For this review, take the finished solid that the model builds, in its own axes (mm). A direction names the side the tool comes from. Round coordinates to 2 decimals unless told otherwise and drop trailing zeros. Order: outer loops, then holes, each group sorted by start corner. A loop starts at its lowest first (then second) coordinate and runs counter-clockwise, first axis right, second up. Notation, with made-up numbers: M -11,11 L 26,11 A24 cw 26,24 Z; hole C 45,63 d4. An arc over 180 degrees is marked long. Use a Markdown table: item, result.
from build123d import *

# Parameters (mm, degrees)
F0_W     = 180.379
F0_H     = 84
F0_W_2   = 176.379
F0_H_2   = 80
F1_DEPTH = 11
F0_W_3   = 164
F0_H_3   = 61
F0_W_4   = 27.5
F0_H_4   = 16
F2_DEPTH = 2
F3_SIZE  = 2


with BuildPart() as f1:
    # F0 (on Top) → F1 (new body)
    with BuildSketch(Plane.XY):
        with Locations((-90.1895, 42)):
            Rectangle(F0_W, F0_H)
        with Locations((-90.1895, 42)):
            Rectangle(F0_W_2, F0_H_2, mode=Mode.SUBTRACT)
    extrude(amount=F1_DEPTH)

    # F0 (on Top) → F2 (join)
    with BuildSketch(Plane.XY):
        with Locations((-90.1895, 42)):
            Rectangle(F0_W_2, F0_H_2)
        with Locations((-91.379, 38.431)):
            Rectangle(F0_W_3, F0_H_3, mode=Mode.SUBTRACT)
        with Locations((-91.379, 38.431)):
            Rectangle(F0_W_3, F0_H_3)
        with BuildLine():
            ThreePointArc((-170.879, 64.931), (-171.9396601718, 67.4916601718), (-169.379, 66.431))
            Line((-169.379, 66.431), (-13.379, 66.431))
            ThreePointArc((-13.379, 66.431), (-11.879, 67.931), (-10.379, 66.431))
            ThreePointArc((-10.379, 66.431), (-10.8183398282, 65.3703398282), (-11.879, 64.931))
            Line((-11.879, 64.931), (-11.879, 11.931))
            ThreePointArc((-11.879, 11.931), (-10.8183398282, 11.4916601718), (-10.379, 10.431))
            ThreePointArc((-10.379, 10.431), (-11.879, 8.931), (-13.379, 10.431))
            Line((-13.379, 10.431), (-169.379, 10.431))
            ThreePointArc((-169.379, 10.431), (-171.9396601718, 9.3703398282), (-170.879, 11.931))
            Line((-170.879, 11.931), (-170.879, 64.931))
        make_face(mode=Mode.SUBTRACT)
        with BuildLine():
            Line((-13.379, 66.431), (-169.379, 66.431))
            ThreePointArc((-169.379, 66.431), (-169.8183398282, 65.3703398282), (-170.879, 64.931))
            Line((-170.879, 64.931), (-170.879, 11.931))
            ThreePointArc((-170.879, 11.931), (-169.8183398282, 11.4916601718), (-169.379, 10.431))
            Line((-169.379, 10.431), (-13.379, 10.431))
            ThreePointArc((-13.379, 10.431), (-12.9396601718, 11.4916601718), (-11.879, 11.931))
            Line((-11.879, 11.931), (-11.879, 64.931))
            ThreePointArc((-11.879, 64.931), (-12.9396601718, 65.3703398282), (-13.379, 66.431))
        make_face()
        with Locations((-119.129, 42.931)):
            Rectangle(F0_W_4, F0_H_4, mode=Mode.SUBTRACT)
    extrude(amount=F2_DEPTH)

    # F3
    f3_edges = [f1.edges().sort_by_distance(p)[0] for p in [
        (0, 42, 0),
        (-90.1895, 84, 0),
        (-90.1895, 0, 0),
        (-180.379, 42, 0),
    ]]
    chamfer(f3_edges, length=F3_SIZE)


solid = f1.part
Q1. Add section A-A (x = -122.5). Write out the cut boundary in (y, z), then the cut area to 3 significant figures.
Determined:
| item | result |
|---|---|
| outline | M 0,2 L 2,0 L 34.93,0 L 34.93,2 L 2,2 L 2,11 L 0,11 Z; M 50.93,0 L 82,0 L 84,2 L 84,11 L 82,11 L 82,2 L 50.93,2 Z |
| area | 168 mm^2 |
Q2. Add section B-B (y = 44). Write out the cut boundary in (x, z).
Determined:
| item | result |
|---|---|
| outline | M -180.38,2 L -178.38,0 L -132.88,0 L -132.88,2 L -178.38,2 L -178.38,11 L -180.38,11 Z; M -105.38,0 L -2,0 L 0,2 L 0,11 L -2,11 L -2,2 L -105.38,2 Z |
Q3. Add section C-C (z = 9). Write out the cut boundary in (x, y).
Determined:
| item | result |
|---|---|
| outline | M -180.38,0 L 0,0 L 0,84 L -180.38,84 Z; hole M -178.38,2 L -2,2 L -2,82 L -178.38,82 Z |
Q4. Add section D-D (y = 7). Write out the cut boundary in (x, z), then the cut area to 3 significant figures.
Determined:
| item | result |
|---|---|
| outline | M -180.38,2 L -178.38,0 L -2,0 L 0,2 L 0,11 L -2,11 L -2,2 L -178.38,2 L -178.38,11 L -180.38,11 Z |
| area | 393 mm^2 |
Q5. Wall thickness on line 1 along X through (y, z) = (36, 4.5); line 2 along Y through (x, z) = (-72, 10); line 3 along Z through (x, y) = (-26, 21): over which ranges is each line inside the solid? List them lowest first. Write a range as [from, to].
Determined:
| item | result |
|---|---|
| line 1 | x = [-180.38, -178.38], [-2, 0] |
| line 2 | y = [0, 2], [82, 84] |
| line 3 | z = [0, 2] |
Q6. Machinability: for faces 4 (the flat face through (-2, 41, 6)), 5 (the flat face through (0, 41, 6)), which of the approach directions +Z, -Z, +X, -X, +Y, -Y give a long, thin tool a straight path to every point of the face, cutting with its end or side? Answer none if there is none.
Determined:
| item | result |
|---|---|
| face 4 | +Z |
| face 5 | +Z, -Z, +X, +Y, -Y |
Q7. Draft analysis for pull direction X (two halves, no side actions). For faces 1 (the flat face through (-178.379, 41, 6)), 2 (the flat face through (-180.379, 41, 6)), 3 (the flat face through (-91, 43, 0)), state which applies: pulls with the +X half, pulls with the -X half, needs draft (parallel to the pull), parting line crosses it, or undercut.
Determined:
| item | result |
|---|---|
| face 1 | undercut |
| face 2 | pulls with the -X half |
| face 3 | needs draft |
Q8. Clearance check with flat-ended pins moving along their axes: pin 1 (2.5 mm diameter, centred on x = -170.879, y = 66.431, fed in from -Z); pin 2 (4 mm diameter, centred on x = -93, y = 36.5, fed in from -Z); pin 3 (0.6 mm diameter, centred on x = -112.5, z = 0.5, fed in from +Y); pin 4 (2 mm diameter, centred on x = -134, y = 59, fed in from +Z). State where each tip first meets the part, or that it passes through.
Determined:
| item | result |
|---|---|
| pin 1 | passes through |
| pin 2 | stops at z = 0 |
| pin 3 | stops at y = 82.8 |
| pin 4 | stops at z = 2 |
